Design review of the part built by this model. Coordinates are the model's own, in mm. A direction names the side the tool comes from. Coordinates: 2 decimals unless noted, no trailing zeros. Write each loop counter-clockwise with the first axis right and the second up, starting at its lowest first coordinate (ties: lowest second). Pieces come first, ordered by that corner, then holes.
Q1. Clearance check with flat-ended pins moving along their axes: pin 1 Ø2 at (y, z) = (-56.5, 15) entering from +X; pin 2 Ø8 at (x, z) = (28.5, 12.5) entering from -Y; pin 3 Ø8 at (x, z) = (18.5, 5) entering from -Y. State where each tip first meets the part, or that it passes through.
Q2. Add section C-C, the plane z = 6. Give the boundary of the cut face in (x, y).
Q3. Add section B-B, the plane y = 0. Give the boundary of the cut face in (x, z), plus the area to 3 significant figures.
Q4. To check wall thickness, follow probe 1 along Y at (x, z) = (-3.5, 16.5); probe 2 along X at (y, z) = (37.5, 2.75); probe 3 along Y at (x, z) = (38.4, 12.5). State the ranges of each line that lie inside material, in increasing order.
Q5. The part is to be moulded in two halves that separate along Z. For faces 1 (the face through (1, 94, 12)), 2 (the face through (29.17, -65.155, 15.173)), 3 (the face through (38, 0, 25)), say which applies: +Z half, -Z half, draft (parallel to the pull), parting line (faces both ways), or undercut.
Q6. Add section D-D, the plane z = 16.5. Give the boundary of the cut face in (x, y).
Q7. Add section A-A, the plane x = -2.5. Give the boundary of the cut face in (y, z), plus the area to 3 significant figures.
Q8. Machinability: for faces 4 (the face through (21.525, 76.369, 20.658)), 5 (the face through (0, 96, 12)), which of the approach directions +Z, -Z, +X, -X, +Y, -Y give a long, thin tool a straight path to every point of the face, cutting with its end or side? Answer none if there is none.
from build123d import *

# Parameters (mm, degrees)
SALIENTE_EXTRUIR2_DEPTH = 25
CROQUIS3_R              = 8.9
CORTAR_EXTRUIR1_DEPTH   = 25
CROQUIS4_R              = 8.9
CORTAR_EXTRUIR2_DEPTH   = 25
CROQUIS5_R              = 8.9
CORTAR_EXTRUIR3_DEPTH   = 25


with BuildPart() as part:
    # Croquis1 → Saliente-Extruir2 (new body)
    with BuildSketch(Plane.XY):
        Polygon((12.5, 96), (39.058112383, 50), (39.058112383, -50), (12.5, -96), (-12.5, -96), (-10.5, -94), (11.345299462, -94), (37.058112383, -49.464101615), (37.058112383, 49.464101615), (11.345299462, 94), (-10.5, 94), (-12.5, 96), align=None)
    extrude(amount=SALIENTE_EXTRUIR2_DEPTH)

    # Croquis3 → Cortar-Extruir1 (cut)
    with BuildSketch(Plane(origin=(39.058112383, 0, 0), x_dir=(0, 0, -1), z_dir=(1, 0, 0))):
        with Locations((-12.5, 0)):
            Circle(CROQUIS3_R)
    extrude(amount=-CORTAR_EXTRUIR1_DEPTH, mode=Mode.SUBTRACT)

    # Croquis4 → Cortar-Extruir2 (cut)
    with BuildSketch(Plane(origin=(50.944219382, 29.412658774, 0), x_dir=(0, 0, -1), z_dir=(0.8660254037844347, 0.500000000000007, 0))):
        with Locations(Location((-12.5, 50.330326381, 0), (0, 0, 90))):
            Circle(CROQUIS4_R)
    extrude(amount=-CORTAR_EXTRUIR2_DEPTH, mode=Mode.SUBTRACT)

    # Croquis5 → Cortar-Extruir3 (cut)
    with BuildSketch(Plane(origin=(50.944219382, -29.412658774, 0), x_dir=(0, 0, -1), z_dir=(0.8660254037844347, -0.500000000000007, 0))):
        with Locations(Location((-12.5, -50.330326381, 0), (0, 0, 90))):
            Circle(CROQUIS5_R)
    extrude(amount=-CORTAR_EXTRUIR3_DEPTH, mode=Mode.SUBTRACT)


solid = part.part
Here are the results:
1. pin 1: stops at x = 35.88
1. pin 2: stops at y = -66.02
1. pin 3: stops at y = -92.54
2. outline: (-12.5, -96) - (12.5, -96) - (22.74, -78.26) - (21.01, -77.26) - (11.35, -94) - (-10.5, -94) - close; (-12.5, 96) - (-10.5, 94) - (11.35, 94) - (21.01, 77.26) - (22.74, 78.26) - (12.5, 96) - close; (27.09, -66.74) - (28.82, -67.74) - (39.06, -50) - (39.06, -6.08) - (37.06, -6.08) - (37.06, -49.46) - close; (27.09, 66.74) - (37.06, 49.46) - (37.06, 6.08) - (39.06, 6.08) - (39.06, 50) - (28.82, 67.74) - close
3. outline: (37.06, 0) - (39.06, 0) - (39.06, 3.6) - (37.06, 3.6) - close; (37.06, 21.4) - (39.06, 21.4) - (39.06, 25) - (37.06, 25) - close
3. area: 14.4 mm2
4. probe 1: y = -96 to -94, 94 to 96
4. probe 2: x = 37.06 to 39.06
4. probe 3: y = -51.14 to -8.9, 8.9 to 51.14
5. face 1: draft
5. face 2: undercut
5. face 3: +Z half
6. outline: (-12.5, -96) - (12.5, -96) - (21.8, -79.89) - (20.07, -78.89) - (11.35, -94) - (-10.5, -94) - close; (-12.5, 96) - (-10.5, 94) - (11.35, 94) - (20.07, 78.89) - (21.8, 79.89) - (12.5, 96) - close; (28.02, -65.11) - (29.75, -66.11) - (39.06, -50) - (39.06, -7.95) - (37.06, -7.95) - (37.06, -49.46) - close; (28.02, 65.11) - (37.06, 49.46) - (37.06, 7.95) - (39.06, 7.95) - (39.06, 50) - (29.75, 66.11) - close
7. outline: (-96, 0) - (-94, 0) - (-94, 25) - (-96, 25) - close; (94, 0) - (96, 0) - (96, 25) - (94, 25) - close
7. area: 100 mm2
8. face 4: +Z, -Z, -X
8. face 5: +Z, -Z, +X, -X, +Y
